```python
from build123d import *

# Parameters (mm, degrees)
SKETCH_1_W          = 40
SKETCH_1_H          = 36
SKETCH_1_R          = 1.6
SKETCH_1_R_2        = 3.25
EXTRUDE_1_DEPTH     = 5
SKETCH_2_R          = 13
CUT_EXTRUDE_1_DEPTH = 2.5
SKETCH_7_R          = 5
EXTRUDE_2_DEPTH     = 10
SKETCH_10_R         = 5
EXTRUDE_4_DEPTH     = 2
EXTRUDE_3_REACH     = 123.4
FILLET_1_R          = 30
FILLET_2_R          = 50
FILLET_6_R          = 5


with BuildPart() as part:
    # ｽｹｯﾁ1 → ﾎﾞｽ - 押し出し1 (new body)
    with BuildSketch(Plane.XY):
        Rectangle(SKETCH_1_W, SKETCH_1_H)
        with Locations((0, 8.5)):
            Circle(SKETCH_1_R, mode=Mode.SUBTRACT)
        with Locations((8.5, 0)):
            Circle(SKETCH_1_R, mode=Mode.SUBTRACT)
        with Locations((0, -8.5)):
            Circle(SKETCH_1_R, mode=Mode.SUBTRACT)
        with Locations((-8.5, 0)):
            Circle(SKETCH_1_R, mode=Mode.SUBTRACT)
        Circle(SKETCH_1_R_2, mode=Mode.SUBTRACT)
    extrude(amount=EXTRUDE_1_DEPTH)

    # ｽｹｯﾁ2 → ｶｯﾄ - 押し出し1 (cut)
    with BuildSketch(Plane.XY.offset(5)):
        Circle(SKETCH_2_R)
    extrude(amount=-CUT_EXTRUDE_1_DEPTH, mode=Mode.SUBTRACT)

    # ｽｹｯﾁ7 → ﾎﾞｽ - 押し出し2 (add)
    with BuildSketch(Plane.XZ.offset(18)):
        Polygon((-20, 0), (-20, 47.190356234), (-7.621741376, 103.02507267), (31.430098909, 94.367488113), (20, 42.809643766), (20, 0), align=None)
        with Locations((0, 45)):
            Circle(SKETCH_7_R, mode=Mode.SUBTRACT)
        with Locations((9.739782627, 88.93332032)):
            Circle(SKETCH_7_R, mode=Mode.SUBTRACT)
    extrude_2 = extrude(amount=EXTRUDE_2_DEPTH)

    # ｽｹｯﾁ10 → ﾎﾞｽ - 押し出し4 (add)
    with BuildSketch(Plane(origin=(0, -18, 0), x_dir=(1, 0, 0), z_dir=(0, 1, 0))):
        with Locations(Location((0, -45, 0), (0, 0, 180))):
            Circle(SKETCH_10_R)
    extrude_4 = extrude(amount=-EXTRUDE_4_DEPTH)

    # ﾐﾗｰ3: ﾎﾞｽ - 押し出し2, ﾎﾞｽ - 押し出し4 across plane
    add(extrude_2.mirror(Plane.ZX))
    add(extrude_4.mirror(Plane.ZX))

    # ﾎﾞｽ - 押し出し3: up to this face of the body (flat: up to its plane)
    extrude_3_end = Plane(part.part.faces().sort_by_distance((-18.848513106, 28, 23.595178117))[0])
    # ｽｹｯﾁ8 → ﾎﾞｽ - 押し出し3 (add, up to the picked face)
    with BuildSketch(Plane.XZ.offset(28), mode=Mode.PRIVATE) as extrude_3_sk1:
        Polygon((-20, 47.190356234), (-20, 0), (-25, 0), (-25, 47.737945292), align=None)
    extrude_3_tool1 = split(extrude(extrude_3_sk1.sketch, amount=-EXTRUDE_3_REACH, mode=Mode.PRIVATE), bisect_by=extrude_3_end, keep=Keep.BOTH, mode=Mode.PRIVATE)
    # ｽｹｯﾁ8 → ﾎﾞｽ - 押し出し3 (add, up to the picked face)
    with BuildSketch(Plane.XZ.offset(28), mode=Mode.PRIVATE) as extrude_3_sk2:
        Polygon((20, 42.809643766), (31.430098909, 94.367488113), (36.311578945, 93.285290043), (25, 42.262054708), (25, 0), (20, 0), align=None)
    extrude_3_tool2 = split(extrude(extrude_3_sk2.sketch, amount=-EXTRUDE_3_REACH, mode=Mode.PRIVATE), bisect_by=extrude_3_end, keep=Keep.BOTH, mode=Mode.PRIVATE)
    add(extrude_3_tool1.solids().sort_by(Axis((-22.504807, -28, 23.732339), (0, 1, 0)))[0])
    add(extrude_3_tool2.solids().sort_by(Axis((25.636945, -28, 47.192298), (0, 1, 0)))[0])

    # ﾌｨﾚｯﾄ1
    # the kernel refuses this fillet: 30 mm, written as the material it adds along each edge
    with BuildSketch(Plane(origin=(-20, 22.088837233, 47.190356234), x_dir=(0.2164396139380964, 0, 0.9762960071199349), z_dir=(0, -1, 0))) as fillet_1_piece_1_section:
        with BuildLine():
            CenterArc((16.035534893, 30), FILLET_1_R, 236.442690238, 33.557309762)
            Line((-0.547589058, 5), (0, 0))
            Line((0, 0), (16.035534893, 0))
        make_face()
    fillet_1_piece_1 = extrude(amount=90.177674467, mode=Mode.PRIVATE)
    fillet_1_piece_1 = split(fillet_1_piece_1, bisect_by=Plane(origin=(-20, 18, 47.190356234), z_dir=(0, 1, 0)), keep=Keep.TOP, mode=Mode.PRIVATE)
    add(fillet_1_piece_1)
    with BuildSketch(Plane(origin=(-20, -18, 47.190356234), x_dir=(0.2164396139380964, 0, 0.9762960071199349), z_dir=(0, -1, 0))) as fillet_1_piece_2:
        with BuildLine():
            CenterArc((16.035534893, 30), FILLET_1_R, 236.442690238, 33.557309762)
            Line((-0.547589058, 5), (0, 0))
            Line((0, 0), (16.035534893, 0))
        make_face()
    extrude(amount=10)
    with BuildSketch(Plane(origin=(-20, -22.088837233, 47.190356234), x_dir=(-0.9940563382222736, 0, 0.10886687485238501), z_dir=(0, 1, 0))) as fillet_1_piece_3_section:
        with BuildLine():
            CenterArc((28.075951576, 19.206231343), FILLET_1_R, 186.25, 33.557309762)
            Line((-1.74573857, 15.940225098), (0, 0))
            Line((0, 0), (5.029896001, 0))
        make_face()
    fillet_1_piece_3 = extrude(amount=90.177674467, mode=Mode.PRIVATE)
    fillet_1_piece_3 = split(fillet_1_piece_3, bisect_by=Plane(origin=(-20, -18, 47.190356234), z_dir=(0, -1, 0)), keep=Keep.TOP, mode=Mode.PRIVATE)
    add(fillet_1_piece_3)
    with BuildSketch(Plane(origin=(-20, 18, 47.190356234), x_dir=(-0.9940563382222736, 0, 0.10886687485238501), z_dir=(0, 1, 0))) as fillet_1_piece_4:
        with BuildLine():
            CenterArc((28.075951576, 19.206231343), FILLET_1_R, 186.25, 33.557309762)
            Line((-1.74573857, 15.940225098), (0, 0))
            Line((0, 0), (5.029896001, 0))
        make_face()
    extrude(amount=10)
    # the kernel refuses this fillet: 30 mm, written as the material it takes off along each edge
    with BuildSketch(Plane(origin=(-7.621741376, 57, 103.02507267), x_dir=(0.9762960071199346, 0, -0.21643961393809735), z_dir=(0, -1, 0))) as fillet_1_2_piece_1:
        with BuildLine():
            CenterArc((FILLET_1_R, -FILLET_1_R), FILLET_1_R, 90, 90)
            Line((0, -FILLET_1_R), (0, 0))
            Line((0, 0), (FILLET_1_R, 0))
        make_face()
    extrude(amount=160, mode=Mode.SUBTRACT)
    with BuildSketch(Plane(origin=(-7.621741376, -57, 103.02507267), x_dir=(0.9762960071199348, 0, -0.21643961393809644), z_dir=(0, 1, 0))) as fillet_1_2_piece_2:
        with BuildLine():
            CenterArc((FILLET_1_R, FILLET_1_R), FILLET_1_R, 180, 90)
            Line((0, FILLET_1_R), (0, 0))
            Line((0, 0), (FILLET_1_R, 0))
        make_face()
    extrude(amount=160, mode=Mode.SUBTRACT)

    # ﾌｨﾚｯﾄ2
    fillet_2_edges = [part.edges().sort_by_distance(p)[0] for p in [
        (25, 0, 42.262054708),
    ]]
    fillet(fillet_2_edges, radius=FILLET_2_R)

    # ﾌｨﾚｯﾄ6
    # the kernel refuses this fillet: 5 mm, written as the material it adds along each edge
    with BuildSketch(Plane(origin=(-7.574295772, 18, 45.829520298), x_dir=(0.10886687485234858, 0, 0.9940563382222776), z_dir=(-0.9940563382222776, 0, 0.1088668748523486))) as fillet_6_piece_1_section:
        with BuildLine():
            CenterArc((FILLET_6_R, -FILLET_6_R), FILLET_6_R, 90, 90)
            Line((0, -FILLET_6_R), (0, 0))
            Line((0, 0), (FILLET_6_R, 0))
        make_face()
    fillet_6_piece_1 = extrude(amount=30.029896001, mode=Mode.PRIVATE)
    fillet_6_piece_1 = split(fillet_6_piece_1, bisect_by=Plane(origin=(-25, 18, 45.829520298), z_dir=(1, 0, 0)), keep=Keep.TOP, mode=Mode.PRIVATE)
    fillet_6_piece_1 = fillet_6_piece_1 - Plane(origin=(-45.818155232, 18, 69.33897334), x_dir=(-0.9940563382223121, 0, 0.10886687485203418), z_dir=(0, -1, 0)) * Cylinder(30, 81, mode=Mode.PRIVATE)
    fillet_6_piece_1 = split(fillet_6_piece_1, bisect_by=Plane(origin=(-20, 18, 45.829520298), z_dir=(-1, 0, 0)), keep=Keep.TOP, mode=Mode.PRIVATE)
    add(fillet_6_piece_1)
    with BuildSketch(Plane(origin=(-37.425704228, -18, 49.098781228), x_dir=(0.10886687485234857, 0, 0.9940563382222776), z_dir=(0.9940563382222777, 0, -0.10886687485234858))) as fillet_6_piece_2_section:
        with BuildLine():
            CenterArc((FILLET_6_R, -FILLET_6_R), FILLET_6_R, 90, 90)
            Line((0, -FILLET_6_R), (0, 0))
            Line((0, 0), (FILLET_6_R, 0))
        make_face()
    fillet_6_piece_2 = extrude(amount=30.029896001, mode=Mode.PRIVATE)
    fillet_6_piece_2 = split(fillet_6_piece_2, bisect_by=Plane(origin=(-25, -18, 49.098781228), z_dir=(1, 0, 0)), keep=Keep.TOP, mode=Mode.PRIVATE)
    fillet_6_piece_2 = split(fillet_6_piece_2, bisect_by=Plane(origin=(-20, -18, 49.098781228), z_dir=(-1, 0, 0)), keep=Keep.TOP, mode=Mode.PRIVATE)
    fillet_6_piece_2 = fillet_6_piece_2 - Plane(origin=(-45.818155232, -18, 69.33897334), x_dir=(0.21643961393799077, 0, 0.9762960071199583), z_dir=(0, 1, 0)) * Cylinder(30, 81, mode=Mode.PRIVATE)
    add(fillet_6_piece_2)


solid = part.part
```
Design review of the part built by this model. Coordinates are the model's own, in mm. A direction names the side the tool comes from. Coordinates: 2 decimals unless noted, no trailing zeros. Loops run counter-clockwise (first coordinate to the right, second up) from the corner with the lowest first, then second, coordinate; pieces in that order, holes last. Notation, with made-up numbers: (26, 16) -> (31, 16) arc R28 ccw to (31, 53) -> close; hole circle Ø1 at (28, 31.5). An arc over 180 degrees is marked (long way). Answer as a JSON object with one key per item and string values.
Q1. Take a section at B-B on x = -0.5. Give the number of separate pieces and of enclosed holes in the cut face, plus the area to 3 significant figures.
Answer block:
{"separate pieces": "4", "enclosed holes": "0", "area": "1,780 mm^2"}
Q2. Take a section at A-A on z = 27.5. Give the boundary of the cut face in (x, y).
Answer block:
{"outline": "(-25, -28) -> (25, -28) -> (25, 28) -> (-25, 28) -> close; hole (-20, -18) -> (20, -18) -> (20, 18) -> (-20, 18) -> close"}
Q3. The part is to be moulded in two halves that separate along Z. For faces 1 (the cylindrical face through (-0.651, -23.944, 49.957)), 2 (the cylindrical face through (12.43, -22.93, 93.15)), 3 (the flat face through (25, 0, 19)), 4 (the flat face through (-22.54, -0.18, 47.47)), say which applies: +Z half, -Z half, draft (parallel to the pull), parting line (faces both ways), or undercut.
Answer block:
{"face 1": "undercut", "face 2": "undercut", "face 3": "draft", "face 4": "+Z half"}
Q4. Take a section at C-C on y = -22.5. Give the boundary of the cut face in (x, z), plus the area to 3 significant figures.
Answer block:
{"outline": "(-25, 0) -> (25, 0) -> (25, 36.79) arc R50 cw to (26.19, 47.61) -> (36.31, 93.29) -> (21.67, 96.53) arc R30 ccw to (-14.11, 73.74) -> (-16.53, 62.85) arc R30 cw to (-25, 47.74) -> close; hole circle Ø10 at (0, 45); hole circle Ø10 at (9.74, 88.93)", "area": "4,390 mm^2"}
Q5. Tool access review of faces 5 (the flat face through (6, 18, 50)), 6 (the flat face through (-15.34, 22.93, 68.21)), 7 (the cylindrical face through (-0.651, 23.944, 49.957)): name each direction out of +Z, -Z, +X, -X, +Y, -Y from which nothing blocks a thin tool from reaching the whole face with its end or side.
Answer block:
{"face 5": "+Z", "face 6": "+Z, -X, +Y, -Y", "face 7": "+Y"}
Q6. To check wall thickness, follow L1, parallel to Y at x = 0, z = 1.75; L2, parallel to X at y = 0, z = 1; L3, parallel to X at y = -5, z = 28.5. State the ranges of each line that lie inside material, in increasing order.
Answer block:
{"L1": "y = -28 to -10.1, -6.9 to -3.25, 3.25 to 6.9, 10.1 to 28", "L2": "x = -25 to -10.1, -6.9 to -3.25, 3.25 to 6.9, 10.1 to 25", "L3": "x = -25 to -20, 20 to 25"}
Q7. Clearance check with flat-ended pins moving along their axes: pin 1 Ø8.5 at (x, y) = (0, 0) entering from +Z; pin 2 Ø10 at (y, z) = (-9.5, 41.5) entering from +X; pin 3 Ø2 at (y, z) = (22, 74) entering from +X. State where each tip first meets the part, or that it passes through.
Answer block:
{"pin 1": "stops at z = 2.5", "pin 2": "stops at x = 25.95", "pin 3": "stops at x = 32.26"}
Q8. Take a section at D-D on x = -8.5. Give the boundary of the cut face in (y, z).
Answer block:
{"outline": "(-28, 0) -> (-1.6, 0) -> (-1.6, 2.5) -> (-9.84, 2.5) -> (-9.84, 5) -> (-18, 5) -> (-18, 85.67) -> (-28, 85.67) -> close; (1.6, 0) -> (28, 0) -> (28, 85.67) -> (18, 85.67) -> (18, 5) -> (9.84, 5) -> (9.84, 2.5) -> (1.6, 2.5) -> close"}
